from build123d import *

# Parameters (mm, degrees)
SKETCH2_W                                       = 120
SKETCH2_H                                       = 50
BOSS_EXTRUDE3_DEPTH                             = 17
SKETCH4_W                                       = 110
SKETCH4_H                                       = 40
CUT_EXTRUDE1_DEPTH                              = 10
CSK_FOR_M3_FLAT_HEAD_MACHINE_SCREW1_D           = 3.4
CSK_FOR_M3_FLAT_HEAD_MACHINE_SCREW1_DEPTH       = 5
CSK_FOR_M3_FLAT_HEAD_MACHINE_SCREW1_CSINK_D     = 6.3
CSK_FOR_M3_FLAT_HEAD_MACHINE_SCREW1_CSINK_ANGLE = 90
CSK_FOR_M4_FLAT_HEAD_MACHINE_SCREW3_D           = 4.5
CSK_FOR_M4_FLAT_HEAD_MACHINE_SCREW3_CSINK_D     = 9.4
CSK_FOR_M4_FLAT_HEAD_MACHINE_SCREW3_CSINK_ANGLE = 90


with BuildPart() as part:
    # Sketch2 → Boss-Extrude3 (new body)
    with BuildSketch(Plane.XY):
        with Locations((60, 25)):
            Rectangle(SKETCH2_W, SKETCH2_H)
    extrude(amount=BOSS_EXTRUDE3_DEPTH)

    # Sketch4 → Cut-Extrude1 (cut)
    with BuildSketch(Plane.XY.offset(17)):
        with Locations((60, 25)):
            Rectangle(SKETCH4_W, SKETCH4_H)
    extrude(amount=-CUT_EXTRUDE1_DEPTH, mode=Mode.SUBTRACT)

    # CSK for M3 Flat Head Machine Screw1
    with Locations(Plane(origin=(0, 45, 0), x_dir=(-1, 0, 0), z_dir=(0, -1, 0))):
        with Locations((-42.5, -12), (-77.5, -12)):
            CounterSinkHole(CSK_FOR_M3_FLAT_HEAD_MACHINE_SCREW1_D / 2, CSK_FOR_M3_FLAT_HEAD_MACHINE_SCREW1_CSINK_D / 2, depth=CSK_FOR_M3_FLAT_HEAD_MACHINE_SCREW1_DEPTH, counter_sink_angle=CSK_FOR_M3_FLAT_HEAD_MACHINE_SCREW1_CSINK_ANGLE)

    # CSK for M4 Flat Head Machine Screw3 (through all)
    with Locations(Plane(origin=(0, 0, 0), x_dir=(-1, 0, 0), z_dir=(0, 0, -1))):
        with Locations((-97.5, 17), (-22.5, 17)):
            CounterSinkHole(CSK_FOR_M4_FLAT_HEAD_MACHINE_SCREW3_D / 2, CSK_FOR_M4_FLAT_HEAD_MACHINE_SCREW3_CSINK_D / 2, counter_sink_angle=CSK_FOR_M4_FLAT_HEAD_MACHINE_SCREW3_CSINK_ANGLE)


solid = part.part
Design review of the part built by this model. Coordinates are the model's own, in mm. A direction names the side the tool comes from. Coordinates: 2 decimals unless noted, no trailing zeros. Loops run counter-clockwise (first coordinate to the right, second up) from the corner with the lowest first, then second, coordinate; pieces in that order, holes last.
Item 1: Draft analysis for pull direction Z (two halves, no side actions). For faces 1 (the flat face through (59, 25, 7)), 2 (the cylindrical face through (41.15, 48.25, 13.03)), 3 (the flat face through (59, 50, 8)), state which applies: pulls with the +Z half, pulls with the -Z half, needs draft (parallel to the pull), parting line crosses it, or undercut.
Completed:
face 1: pulls with the +Z half
face 2: undercut
face 3: needs draft
Item 2: Wall thickness on L1, parallel to X at y = 17, z = 4.8; L2, parallel to Y at x = 39.5, z = 7.5; L3, parallel to X at y = 33, z = 11.5: over which ranges is each line inside the solid? List them lowest first.
Completed:
L1: x = 0 to 20.25, 24.75 to 95.25, 99.75 to 120
L2: y = 0 to 5, 45 to 50
L3: x = 0 to 5, 115 to 120
Item 3: Add section C-C (x = 97.5). Write out the cut boundary in (y, z).
Completed:
outline: (0, 0) - (12.3, 0) - (14.75, 2.45) - (14.75, 7) - (5, 7) - (5, 17) - (0, 17) - close; (19.25, 2.45) - (21.7, 0) - (50, 0) - (50, 17) - (45, 17) - (45, 7) - (19.25, 7) - close
Item 4: Add section A-A (y = 17). Write out the cut boundary in (x, z), and give its area (3 significant figures).
Completed:
outline: (0, 0) - (17.8, 0) - (20.25, 2.45) - (20.25, 7) - (5, 7) - (5, 17) - (0, 17) - close; (24.75, 2.45) - (27.2, 0) - (92.8, 0) - (95.25, 2.45) - (95.25, 7) - (24.75, 7) - close; (99.75, 2.45) - (102.2, 0) - (120, 0) - (120, 17) - (115, 17) - (115, 7) - (99.75, 7) - close
area: 865 mm2
Item 5: Add section B-B (z = 12). Write out the cut boundary in (x, y).
Completed:
outline: (0, 0) - (120, 0) - (120, 50) - (79.2, 50) - (79.2, 46.45) - (80.65, 45) - (115, 45) - (115, 5) - (5, 5) - (5, 45) - (39.35, 45) - (40.8, 46.45) - (40.8, 50) - (0, 50) - close; (44.2, 46.45) - (45.65, 45) - (74.35, 45) - (75.8, 46.45) - (75.8, 50) - (44.2, 50) - close
Item 6: Clearance check with flat-ended pins moving along their axes: pin 1 (3.5 mm diameter, centred on x = 97.5, y = 17, fed in from +Z); pin 2 (7 mm diameter, centred on x = 22.5, y = 17, fed in from +Z); pin 3 (2 mm diameter, centred on x = 42.5, z = 12, fed in from +Y). State where each tip first meets the part, or that it passes through.
Completed:
pin 1: passes through
pin 2: stops at z = 7
pin 3: stops at y = 5
Item 7: For faces 4 (the flat face through (115, 25, 12)), 5 (the cylindrical face through (23.538, 15.004, 4.757)), 6 (the cylindrical face through (75.8, 48.25, 11.93)), list the 3-axis set-ups (+Z, -Z, +X, -X, +Y, -Y) from which the entire face can be reached by the end or side of a thin tool; tool diameter is ignored.
Completed:
face 4: +Z
face 5: +Z, -Z
face 6: +Y
Item 8: Add section D-D (x = 35). Write out the cut boundary in (y, z), and give its area (3 significant figures).
Completed:
outline: (0, 0) - (50, 0) - (50, 17) - (45, 17) - (45, 7) - (5, 7) - (5, 17) - (0, 17) - close
area: 450 mm2
